For this review, use the dimensioned drawing (mm, ordinates from the lowest corner) and the shaded views. Coordinates: 2 decimals unless noted, no trailing zeros. Order: outer loops, then holes, each group sorted by start corner. A loop starts at its lowest first (then second) coordinate and runs counter-clockwise, first axis right, second up. Notation, with made-up numbers: M -24,-34 L -9,-34 A13 cw -9,-24 Z; hole C 13.25,16.25 d2. An arc over 180 degrees is marked long. Write each question's results on one line, items separated by ' | '.
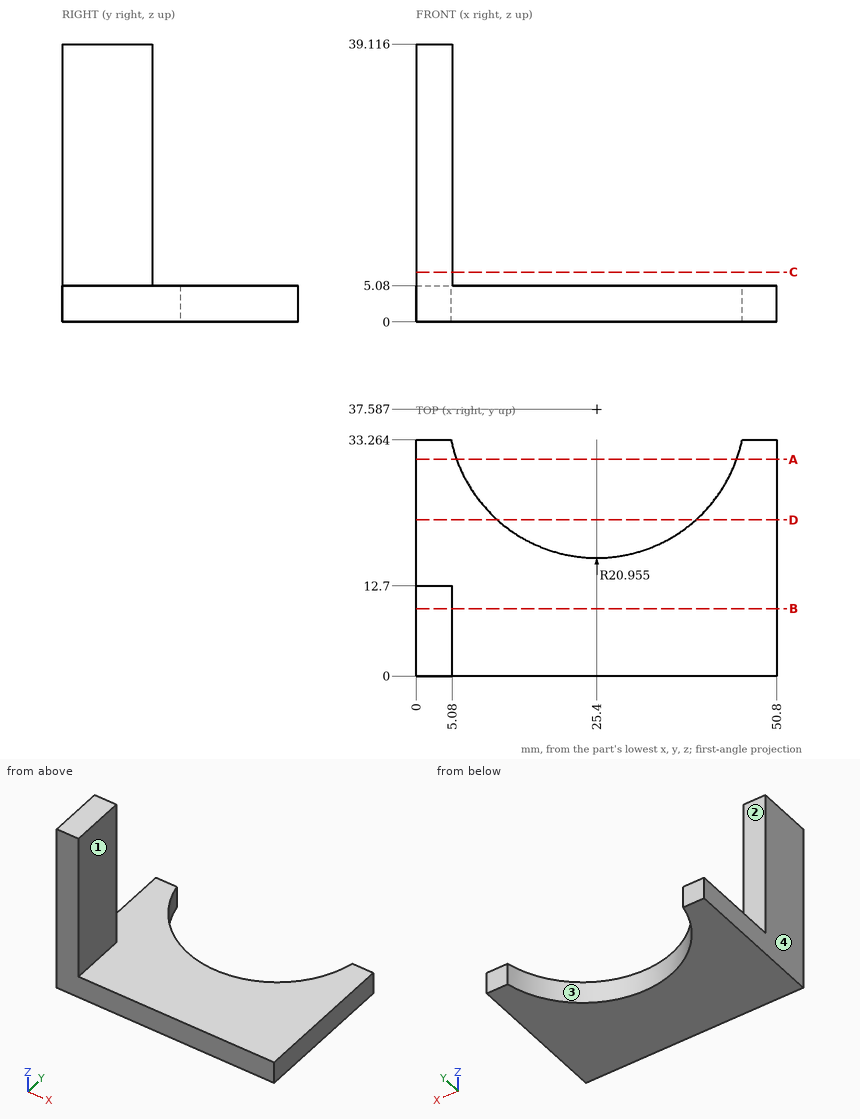
1) Take a section at C-C on z = 7. State the section outline as (x, y) points.
Solutions:
outline: M 0,0 L 5.08,0 L 5.08,12.7 L 0,12.7 Z
2) For pin 1 (14 mm diameter, centred on y = 7, z = 24, fed in from +X); pin 2 (2.5 mm diameter, centred on x = 1.5, z = 25.5, fed in from +Y); pin 3 (16.5 mm diameter, centred on x = 21, y = 17.5, fed in from +Z); pin 4 (1 mm diameter, centred on y = 13.5, z = 21, fed in from -X), all flat-tipped, find the tip position at first contact; note any pin that passes through.
Solutions:
pin 1: x = 5.08 | pin 2: y = 12.7 | pin 3: z = 5.08 | pin 4: through
3) Take a section at A-A on y = 30.5. State the section outline as (x, z) points, plus the area to 3 significant figures.
Solutions:
outline: M 0,0 L 5.68,0 L 5.68,5.08 L 0,5.08 Z; M 45.12,0 L 50.8,0 L 50.8,5.08 L 45.12,5.08 Z | area: 57.7 mm2
4) The part is to be moulded in two halves that separate along X. For the marked faces 1, 2, 3 and 4, say which applies: pulls with the +X half, pulls with the -X half, needs draft (parallel to the pull), parting line crosses it, or undercut.
Solutions:
face 1: pulls with the +X half | face 2: needs draft | face 3: undercut | face 4: pulls with the -X half
5) Take a section at B-B on y = 9.5. State the section outline as (x, z) points.
Solutions:
outline: M 0,0 L 50.8,0 L 50.8,5.08 L 5.08,5.08 L 5.08,39.12 L 0,39.12 Z
6) Take a section at D-D on y = 22. State the section outline as (x, z) points, plus the area to 3 significant figures.
Solutions:
outline: M 0,0 L 11.39,0 L 11.39,5.08 L 0,5.08 Z; M 39.41,0 L 50.8,0 L 50.8,5.08 L 39.41,5.08 Z | area: 116 mm2
7) To check wall thickness, follow line 1 along Z through (x, y) = (28, 10); line 2 along X through (y, z) = (23.5, 4). State the ranges of each line that lie inside material, in increasing order.
Solutions:
line 1: 0 to 5.08 | line 2: 0 to 9.89, 40.91 to 50.8
